```python
from build123d import *

# Parameters (mm, degrees)
SKETCH_1_R          = 30
EXTRUDE_1_DEPTH     = 5
SKETCH_2_W          = 20
SKETCH_2_H          = 20
EXTRUDE_2_DEPTH     = 30
EXTRUDE_START       = 5
SKETCH_4_R          = 30
EXTRUDE_3_DEPTH     = 5
CUT_EXTRUDE_1_DEPTH = 30
SKETCH_7_R          = 2.1
CUT_EXTRUDE_2_DEPTH = 30
SKETCH_8_R          = 3.5
CUT_EXTRUDE_3_DEPTH = 5


with BuildPart() as part:
    # 草图1 → 凸台-拉伸1 (new body)
    with BuildSketch(Plane(origin=(0, 0, 0), x_dir=(0, 0, -1), z_dir=(1, 0, 0))):
        Circle(SKETCH_1_R)
    extrude(amount=EXTRUDE_1_DEPTH)

    # 草图2 → 凸台-拉伸2 (add)
    with BuildSketch(Plane(origin=(5, 0, 0), x_dir=(0, 0, -1), z_dir=(1, 0, 0))):
        Rectangle(SKETCH_2_W, SKETCH_2_H)
    extrude(amount=EXTRUDE_2_DEPTH)

    # 草图4 → 凸台-拉伸3 (add)
    with BuildSketch(Plane.ZY.offset(EXTRUDE_START)):
        Circle(SKETCH_4_R)
    extrude(amount=-EXTRUDE_3_DEPTH)

    # 草图5 → 切除-拉伸1 (cut)
    with BuildSketch(Plane(origin=(35, 0, 0), x_dir=(0, 0, -1), z_dir=(1, 0, 0))):
        Polygon((-10, 3), (-10, 0), (-4, 0), (-4, 3), (-6.5, 5.5), (-8.5, 5.5), (-8.5, 3), align=None)
        Polygon((-4, 0), (-10, 0), (-10, -3), (-8.5, -3), (-8.5, -5.5), (-6.5, -5.5), (-4, -3), align=None)
        Polygon((-3, -8.5), (-3, -10), (3, -10), (3, -8.5), (5.5, -8.5), (5.5, -6.5), (3, -4), (-3, -4), (-5.5, -6.5), (-5.5, -8.5), align=None)
        Polygon((10, -3), (10, 3), (8.5, 3), (8.5, 5.5), (6.5, 5.5), (4, 3), (4, -3), (6.5, -5.5), (8.5, -5.5), (8.5, -3), align=None)
        Polygon((3, 10), (-3, 10), (-3, 8.5), (-5.5, 8.5), (-5.5, 6.5), (-3, 4), (3, 4), (5.5, 6.5), (5.5, 8.5), (3, 8.5), align=None)
    extrude(amount=-CUT_EXTRUDE_1_DEPTH, mode=Mode.SUBTRACT)

    # 草图7 → 切除-拉伸2 (cut)
    with BuildSketch(Plane.ZY.offset(5)):
        with Locations((0, -17.25)):
            Circle(SKETCH_7_R)
        with Locations((-14.938938215, -8.625)):
            Circle(SKETCH_7_R)
        with Locations((-14.938938215, 8.625)):
            Circle(SKETCH_7_R)
        with Locations((0, 17.25)):
            Circle(SKETCH_7_R)
        with Locations((14.938938215, 8.625)):
            Circle(SKETCH_7_R)
        with Locations((14.938938215, -8.625)):
            Circle(SKETCH_7_R)
    extrude(amount=-CUT_EXTRUDE_2_DEPTH, mode=Mode.SUBTRACT)

    # 草图8 → 切除-拉伸3 (cut)
    with BuildSketch(Plane(origin=(5, 0, 0), x_dir=(0, 0, -1), z_dir=(1, 0, 0))):
        with Locations((-14.938938215, 8.625)):
            Circle(SKETCH_8_R)
        with Locations((0, 17.25)):
            Circle(SKETCH_8_R)
        with Locations((14.938938215, 8.625)):
            Circle(SKETCH_8_R)
        with Locations((14.938938215, -8.625)):
            Circle(SKETCH_8_R)
        with Locations((0, -17.25)):
            Circle(SKETCH_8_R)
        with Locations((-14.938938215, -8.625)):
            Circle(SKETCH_8_R)
    extrude(amount=-CUT_EXTRUDE_3_DEPTH, mode=Mode.SUBTRACT)


solid = part.part
```
Geometry check sheet. Reference: the model listing, model coordinates, mm. A direction names the side the tool comes from. Round coordinates to 2 decimals unless told otherwise and drop trailing zeros. Order: outer loops, then holes, each group sorted by start corner. A loop starts at its lowest first (then second) coordinate and runs counter-clockwise, first axis right, second up. Notation, with made-up numbers: (20, 45.25) -> (57, 45.25) arc R34 cw to (57, 76.25) -> close; hole circle Ø4 at (-18.5, -31.75). An arc over 180 degrees is marked (long way). Return JSON: item names as keys, results as strings. Group by question number.
Q1. Tool access check on faces 4 (the flat face through (20, 6, -10)), 5 (the flat face through (20, 3, 9)), 6 (the flat face through (20, -10, 7)), 7 (the flat face through (20, 7, -5.5)), 8 (the flat face through (20, -4, 0)). Record the directions out of +Z, -Z, +X, -X, +Y, -Y that give a thin tool (end or side, any length) a straight path to the whole face; none if there is none.
Q2. Section check A-A, the plane y = 16. Record the boundary of the cut face in (x, z).
Q3. Section check C-C, the plane y = 0. Record the boundary of the cut face in (x, z), plus the area to 3 significant figures.
Q4. Section check D-D, the plane z = -7.5. Record the boundary of the cut face in (x, y), plus the area to 3 significant figures.
Q5. Material ranges on probe 1 along Y at (x, z) = (-3, 0); probe 2 along Y at (x, z) = (19.5, -6); probe 3 along Y at (x, z) = (1.75, 0), recorded low to high. Write a range as from..to.
Q6. Gauge pin test, flat ends, axial feed: pin 1 (5 mm diameter, centred on x = 3.5, y = 12, fed in from +Z); pin 2 (1.6 mm diameter, centred on x = 25.5, z = 8, fed in from -Y); pin 3 (8 mm diameter, centred on y = 8.62, z = -14.94, fed in from +X); pin 4 (3.5 mm diameter, centred on y = 8.62, z = -14.94, fed in from +X). Record the tip position at first contact, or that the pin passes through.
Q7. Release check for a two-part mould opening along Z. For faces 1 (the flat face through (20, 8.5, -4)), 2 (the flat face through (20, -7, 10)), 3 (the flat face through (20, -3, -9)) record: released by +Z, released by -Z, zero draft, split by the parting line, or undercut.
Q8. Section check B-B, the plane z = 0. Record the boundary of the cut face in (x, y).
Numbers:
{
 "1": {"face 4": "-Z, +X, +Y, -Y", "face 5": "+Z, +X", "face 6": "+Z, -Z, +X, -Y", "face 7": "+X", "face 8": "+X, -Y"},
 "2": {"outline": "(-5, -25.38) -> (5, -25.38) -> (5, -3.27) -> (0, -3.27) -> (0, -1.69) -> (-5, -1.69) -> close; (-5, 1.69) -> (0, 1.69) -> (0, 3.27) -> (5, 3.27) -> (5, 25.38) -> (-5, 25.38) -> close"},
 "3": {"outline": "(-5, -30) -> (5, -30) -> (5, -4) -> (35, -4) -> (35, 4) -> (5, 4) -> (5, 30) -> (-5, 30) -> close", "area": "840 mm^2"},
 "4": {"outline": "(-5, -29.05) -> (5, -29.05) -> (5, -10) -> (35, -10) -> (35, -5.5) -> (5, -5.5) -> (5, 5.5) -> (35, 5.5) -> (35, 10) -> (5, 10) -> (5, 29.05) -> (-5, 29.05) -> close", "area": "851 mm^2"},
 "5": {"probe 1": "-30..-19.35, -15.15..15.15, 19.35..30", "probe 2": "-10..-5, 5..10", "probe 3": "-30..-20.75, -13.75..13.75, 20.75..30"},
 "6": {"pin 1": "z = 28.46", "pin 2": "y = -10", "pin 3": "x = 5", "pin 4": "through"},
 "7": {"face 1": "undercut", "face 2": "released by +Z", "face 3": "zero draft"},
 "8": {"outline": "(-5, -30) -> (5, -30) -> (5, -20.75) -> (0, -20.75) -> (0, -19.35) -> (-5, -19.35) -> close; (-5, -15.15) -> (0, -15.15) -> (0, -13.75) -> (5, -13.75) -> (5, -4) -> (35, -4) -> (35, 4) -> (5, 4) -> (5, 13.75) -> (0, 13.75) -> (0, 15.15) -> (-5, 15.15) -> close; (-5, 19.35) -> (0, 19.35) -> (0, 20.75) -> (5, 20.75) -> (5, 30) -> (-5, 30) -> close"}
}
